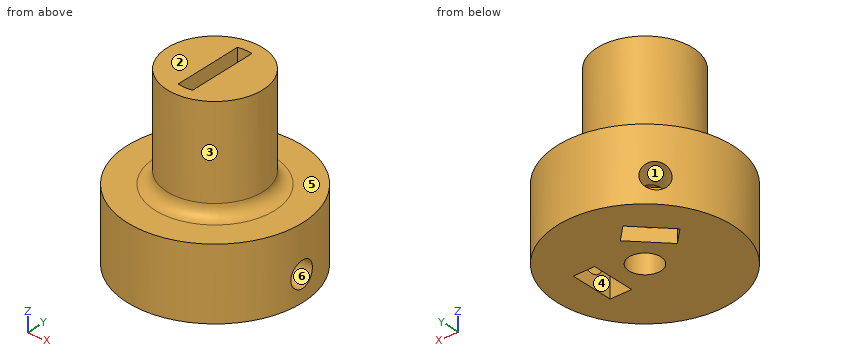
```python
from build123d import *

# Parameters (mm, degrees)
SKETCH1_R           = 6
SKETCH1_R_2         = 2
BOSS_EXTRUDE1_DEPTH = 9
SKETCH2_R           = 6
BOSS_EXTRUDE2_DEPTH = 3
BOSS_EXTRUDE3_DEPTH = 10
SKETCH4_R           = 6
SKETCH4_R_2         = 4.5
BOSS_EXTRUDE4_DEPTH = 10
BOSS_EXTRUDE5_START = 9
SKETCH5_R           = 11
SKETCH5_R_2         = 6
BOSS_EXTRUDE5_DEPTH = 9
SKETCH6_W           = 2.7
SKETCH6_H           = 5.5
CUT_EXTRUDE1_DEPTH  = 6.2
SKETCH7_R           = 1.6
CUT_EXTRUDE2_DEPTH  = 29.809720582
SKETCH8_R           = 1.6
CUT_EXTRUDE3_DEPTH  = 30.43544272
FILLET1_R           = 0.9
FILLET2_R           = 1.5


with BuildPart() as part:
    # Sketch1 → Boss-Extrude1 (new body)
    with BuildSketch(Plane.XY):
        Circle(SKETCH1_R)
        Circle(SKETCH1_R_2, mode=Mode.SUBTRACT)
    extrude(amount=BOSS_EXTRUDE1_DEPTH)

    # Sketch2 → Boss-Extrude2 (add)
    with BuildSketch(Plane.XY.offset(9)):
        Circle(SKETCH2_R)
    extrude(amount=BOSS_EXTRUDE2_DEPTH)

    # Sketch3 → Boss-Extrude3 (add)
    with BuildSketch(Plane.XY.offset(12)):
        with BuildLine():
            Line((0.9, 4.409081537), (0.9, -4.409081537))
            ThreePointArc((0.9, -4.409081537), (4.5, 0), (0.9, 4.409081537))
        make_face()
        with BuildLine():
            Line((-0.9, 4.409081537), (-0.9, -4.409081537))
            ThreePointArc((-0.9, -4.409081537), (-4.5, 0), (-0.9, 4.409081537))
        make_face()
    extrude(amount=BOSS_EXTRUDE3_DEPTH)

    # Sketch4 → Boss-Extrude4 (add)
    with BuildSketch(Plane.XY.offset(12)):
        Circle(SKETCH4_R)
        Circle(SKETCH4_R_2, mode=Mode.SUBTRACT)
    extrude(amount=BOSS_EXTRUDE4_DEPTH)

    # Sketch5 → Boss-Extrude5 (add)
    with BuildSketch(Plane(origin=(0, 0, 9), x_dir=(-1, 0, 0), z_dir=(0, 0, -1)).offset(BOSS_EXTRUDE5_START)):
        with Locations(Location((0, 0, 0), (0, 0, 180))):
            Circle(SKETCH5_R)
        Circle(SKETCH5_R_2, mode=Mode.SUBTRACT)
    extrude(amount=-BOSS_EXTRUDE5_DEPTH)

    # Sketch6 → Cut-Extrude1 (cut)
    with BuildSketch(Plane(origin=(0, 0, 0), x_dir=(-1, 0, 0), z_dir=(0, 0, -1))):
        with Locations((-5.35, 0)):
            Rectangle(SKETCH6_W, SKETCH6_H)
        Polygon((2.855831889, 6.655578529), (6.708147842, 2.730064321), (4.781077231, 0.838927398), (0.928761278, 4.764441606), align=None)
    extrude(amount=-CUT_EXTRUDE1_DEPTH, mode=Mode.SUBTRACT)

    # Sketch7 → Cut-Extrude2 (cut, through all)
    with BuildSketch(Plane(origin=(4, 0, 0), x_dir=(0, 0, -1), z_dir=(1, 0, 0))):
        with Locations((-3.2, 0)):
            Circle(SKETCH7_R)
    extrude(amount=CUT_EXTRUDE2_DEPTH, mode=Mode.SUBTRACT)

    # Sketch8 → Cut-Extrude3 (cut, through all)
    with BuildSketch(Plane(origin=(-2.854919424, 2.80168433, 0), x_dir=(0, 0, 1), z_dir=(-0.7137298559492212, 0.7004210824402017, 0))):
        with Locations(Location((3.2, 0, 0), (0, 0, 90))):
            Circle(SKETCH8_R)
    extrude(amount=CUT_EXTRUDE3_DEPTH, mode=Mode.SUBTRACT)

    # Fillet1
    fillet1_edges = [part.edges().sort_by_distance(p)[0] for p in [
        (0.9, 0, 12),
        (-0.9, 0, 12),
        (0, 4.5, 12),
        (0, -4.5, 12),
    ]]
    fillet(fillet1_edges, radius=FILLET1_R - 0.0001)  # a hair under: the kernel refuses the full size

    # Fillet2
    fillet2_edges = [part.edges().sort_by_distance(p)[0] for p in [
        (-6, 0, 9),
    ]]
    fillet(fillet2_edges, radius=FILLET2_R)


solid = part.part
```
Can you work these out from the model? Positions are in its coordinate system, mm. Face numbers are marked on the shaded views. A direction names the side the tool comes from. Round coordinates to 2 decimals unless told otherwise and drop trailing zeros. Loops run counter-clockwise (first coordinate to the right, second up) from the corner with the lowest first, then second, coordinate; pieces in that order, holes last. Notation, with made-up numbers: (12.5, -15.75) -> (16.5, -15.75) arc R27 cw to (16.5, 19.25) -> close; hole circle Ø7 at (55.25, 40.25). An arc over 180 degrees is marked (long way). One line per item, written item: value. Start each with the question number.
1. For pin 1 (6 mm diameter, centred on y = -3.5, z = 6, fed in from +X); pin 2 (1 mm diameter, centred on y = 2.5, z = 8.5, fed in from +X); pin 3 (6 mm diameter, centred on x = -1, z = 6, fed in from +Y); pin 4 (2.5 mm diameter, centred on y = -1, z = 19.5, fed in from +X), each with a flat end and sliding along its axis, tell me the tip position at first contact or that it passes through.
2. For the marked faces 4, 5 and 6, which set-ups out of +Z, -Z, +X, -X, +Y, -Y let a thin tool reach every point of the face, with its end or its side?
3. If we section it at D-D, the plane z = 4.25: Write out the boundary of the cut face in (x, y), then the cut area to 3 significant figures.
4. If we section it at C-C, the plane x = 8.75: Write out the boundary of the cut face in (y, z).
5. If we section it at B-B, the plane z = 18: Write out the boundary of the cut face in (x, y), then the cut area to 3 significant figures.
6. If I drill on probe 1 along Y at (x, z) = (0, 7); probe 2 along Z at (x, y) = (-3.25, 4.75); probe 3 along Z at (x, y) = (-6.25, -4.25), over which ranges is the centre line in solid material (lowest first)?
7. If we mould it in two halves opening along Y, with no side actions, what happens to the marked faces 1, 2 and 3? For each: pulls with the +Y half, pulls with the -Y half, needs draft (parallel to the pull), parting line crosses it, or undercut.
Calculated:
1. pin 1: stops at x = 10.99
1. pin 2: stops at x = 10.82
1. pin 3: stops at y = 11
1. pin 4: stops at x = 6
2. face 4: -Z
2. face 5: +Z
2. face 6: +X
3. outline: (-8.65, 6.8) arc R11 ccw (long way) to (10.93, -1.21) -> (6.7, -1.21) -> (6.7, -2.75) -> (4, -2.75) -> (4, 2.75) -> (6.7, 2.75) -> (6.7, 1.21) -> (10.93, 1.21) arc R11 ccw to (-6.96, 8.52) -> (-3.94, 5.55) -> (-2.86, 6.66) -> (-0.93, 4.76) -> (-4.78, 0.84) -> (-6.71, 2.73) -> (-5.63, 3.83) -> close; hole circle Ø4 at (0, 0)
3. area: 317 mm²
4. outline: (-6.67, 0) -> (6.67, 0) -> (6.67, 9) -> (-6.67, 9) -> close; hole circle Ø3.2 at (0, 3.2)
5. outline: circle Ø12 at (0, 0); hole (-0.9, -4.41) arc R4.5 ccw to (0.9, -4.41) -> (0.9, 4.41) arc R4.5 ccw to (-0.9, 4.41) -> close
5. area: 97.0 mm²
6. probe 1: y = -11 to -2, 2 to 11
6. probe 2: z = 6.2 to 22
6. probe 3: z = 0 to 9
7. face 1: undercut
7. face 2: needs draft
7. face 3: parting line crosses it
